Source: three-view drawing plus pictorial views. Frame: mm from the lowest corner of the part. A direction names the side the tool comes from. Give positions to 0.01 mm unless a question says otherwise; leave off trailing zeros. Loops run counter-clockwise (first coordinate to the right, second up) from the corner with the lowest first, then second, coordinate; pieces in that order, holes last. Notation, with made-up numbers: (-13, 35.5) -> (19, 35.5) arc R26 cw to (19, 69.5) -> close; hole circle Ø11 at (-17, 1.5). An arc over 180 degrees is marked (long way). One line per item, written item: value. Start each with the question number.
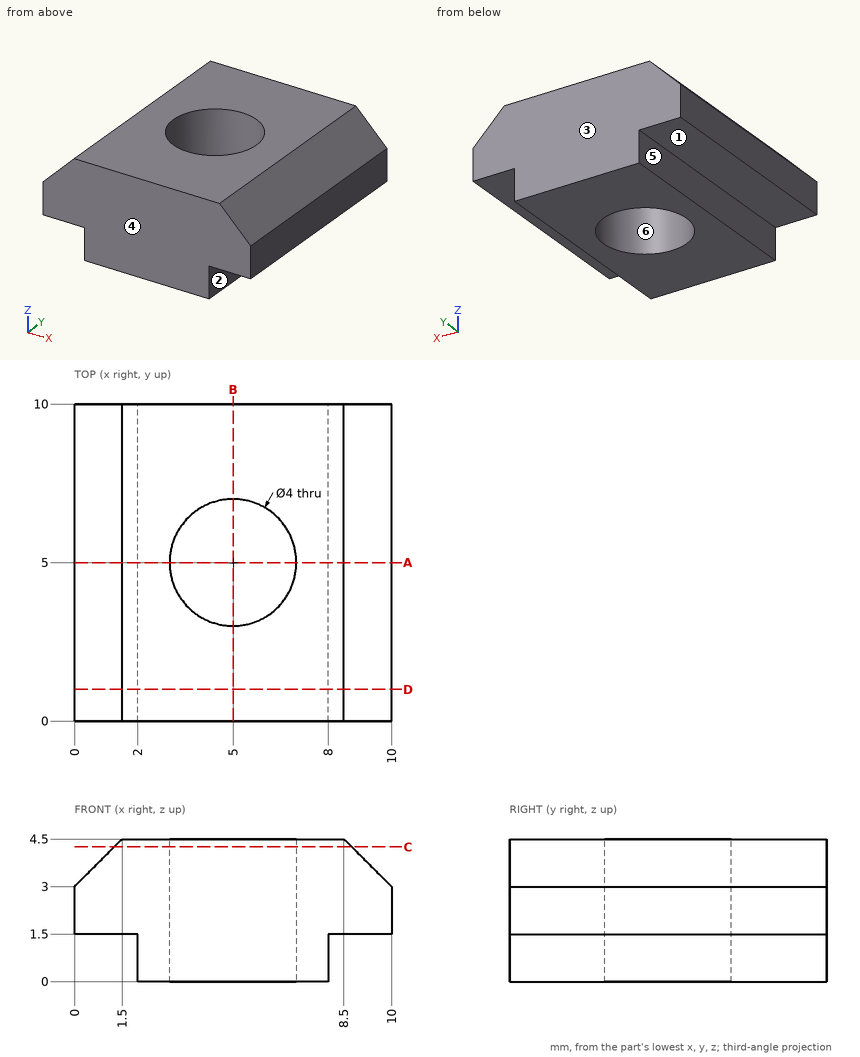
Item 1: Section A-A, the plane y = 5. Output: boundary loops of the cut face in (x, z), then the cut area to 4 significant figures.
Item 2: Ray query, line 1 along Y through (x, z) = (5, 1.7); line 2 along X through (y, z) = (7.75, 0.65); line 3 along Y through (x, z) = (4, 1.85). Return the intervals inside material, ascending. Write a range as [from, to].
Item 3: Pin query (flat end, axial travel): pin 1 (5 mm diameter, centred on x = 5, y = 5, fed in from +Z); pin 2 (2 mm diameter, centred on x = 9.5, y = 7, fed in from -Z); pin 3 (0.8 mm diameter, centred on y = 4.5, z = 1, fed in from +X). Return the tip coordinate at first contact, or that it passes through.
Item 4: Section B-B, the plane x = 5. Output: boundary loops of the cut face in (y, z), then the cut area to 3 significant figures.
Item 5: Access query for the marked faces 1, 2 and 3. Directions: +Z, -Z, +X, -X, +Y, -Y. A direction counts if a zero-diameter tool reaches every point of the face in a straight line with its end or side. Return the directions, or none.
Item 6: Section D-D, the plane y = 1. Output: boundary loops of the cut face in (x, z).
Item 7: Mould query, pull axis Y, two halves, no side actions, for the marked faces 4, 5 and 6. Classes: pulls with the +Y half, pulls with the -Y half, needs draft (parallel to the pull), parting line crosses it, or undercut.
Item 8: Section C-C, the plane z = 4.25. Output: boundary loops of the cut face in (x, y).
Geometry check:
1. outline: (0, 1.5) -> (2, 1.5) -> (2, 0) -> (3, 0) -> (3, 4.5) -> (1.5, 4.5) -> (0, 3) -> close; (7, 0) -> (8, 0) -> (8, 1.5) -> (10, 1.5) -> (10, 3) -> (8.5, 4.5) -> (7, 4.5) -> close
1. area: 18.75 mm2
2. line 1: y = [0, 3], [7, 10]
2. line 2: x = [2, 8]
2. line 3: y = [0, 3.27], [6.73, 10]
3. pin 1: stops at z = 4.5
3. pin 2: stops at z = 1.5
3. pin 3: stops at x = 8
4. outline: (0, 0) -> (3, 0) -> (3, 4.5) -> (0, 4.5) -> close; (7, 0) -> (10, 0) -> (10, 4.5) -> (7, 4.5) -> close
4. area: 27.0 mm2
5. face 1: -Z, -X, +Y, -Y
5. face 2: -Z, +X, +Y, -Y
5. face 3: +Z, -Z, +X, -X, +Y
6. outline: (0, 1.5) -> (2, 1.5) -> (2, 0) -> (8, 0) -> (8, 1.5) -> (10, 1.5) -> (10, 3) -> (8.5, 4.5) -> (1.5, 4.5) -> (0, 3) -> close
7. face 4: pulls with the -Y half
7. face 5: needs draft
7. face 6: undercut
8. outline: (1.25, 0) -> (8.75, 0) -> (8.75, 10) -> (1.25, 10) -> close; hole circle Ø4 at (5, 5)
